Build history of the part. All positions in model axes, mm. A direction names the side the tool comes from. Round coordinates to 2 decimals unless told otherwise and drop trailing zeros. Write each loop counter-clockwise with the first axis right and the second up, starting at its lowest first coordinate (ties: lowest second). Pieces come first, ordered by that corner, then holes. Notation, with made-up numbers: M 7.5,57 L 39.5,57 A23 cw 39.5,81 Z; hole C 52,-35.75 d4. An arc over 180 degrees is marked long. Write item = value, one per line.
from build123d import *

# Parameters (mm, degrees)
PAD_DEPTH       = 20
SKETCH001_R     = 13
POCKET_DEPTH    = 18
SKETCH002_R     = 2.75
POCKET001_DEPTH = 74.863063
POCKET002_START = -20
SKETCH003_R     = 5
POCKET002_DEPTH = 50


with BuildPart() as part:
    # Sketch → Pad (new body)
    with BuildSketch(Plane.XY):
        with BuildLine():
            Line((0, 0), (0, 15))
            Line((24.254781, 65), (0, 15))
            ThreePointArc((55.745219, 65), (40, 74.862063), (24.254781, 65))
            Line((55.745219, 65), (80, 15))
            Line((80, 0), (80, 15))
            Line((0, 0), (80, 0))
        make_face()
    extrude(amount=PAD_DEPTH)

    # Sketch001 (on Face8 of Pad) → Pocket (cut)
    with BuildSketch(Plane.XY.offset(20)):
        with Locations((40, 57.362063)):
            Circle(SKETCH001_R)
    extrude(amount=-POCKET_DEPTH, mode=Mode.SUBTRACT)

    # Sketch002 (on Face7 of Pocket) → Pocket001 (cut, through all)
    with BuildSketch(Plane.XZ):
        with Locations((10, 10)):
            Circle(SKETCH002_R)
        with Locations((70, 10)):
            Circle(SKETCH002_R)
    extrude(amount=-POCKET001_DEPTH, mode=Mode.SUBTRACT)

    # Sketch003 → Pocket002 (cut)
    with BuildSketch(Plane.XZ.offset(POCKET002_START)):
        with Locations((70, 10)):
            Circle(SKETCH003_R)
        with Locations((10, 10)):
            Circle(SKETCH003_R)
    extrude(amount=-POCKET002_DEPTH, mode=Mode.SUBTRACT)


solid = part.part
1. Band-saw the part on D-D (x = 10). List the corners of the cut face in (y, z).
Responses:
outline = M 0,0 L 35.61,0 L 35.61,5 L 20,5 L 20,7.25 L 0,7.25 Z; M 0,12.75 L 20,12.75 L 20,15 L 35.61,15 L 35.61,20 L 0,20 Z
2. Mould opens along X. For faces 4 (the face through (0, 7, 10)), 5 (the face through (39, 0, 10)), 6 (the face through (65, 30, 10)) say: pulls with the +X half, pulls with the -X half, needs draft (parallel to the pull), parting line crosses it, or undercut.
Responses:
face_4 = pulls with the -X half
face_5 = needs draft
face_6 = undercut
3. Band-saw the part on B-B (x = 40). List the corners of the cut face in (y, z), plus the area to 3 significant figures.
Responses:
outline = M 0,0 L 74.86,0 L 74.86,20 L 70.36,20 L 70.36,2 L 44.36,2 L 44.36,20 L 0,20 Z
area = 1,030 mm²
4. Flat gauge pins, fed straight in: pin 1 (5 mm diameter, centred on y = 21.5, z = 5.5, fed in from -X); pin 2 (8 mm diameter, centred on y = 17, z = 6.5, fed in from +X); pin 3 (21 mm diameter, centred on x = 39.5, y = 59.5, fed in from +Z); pin 4 (1.5 mm diameter, centred on y = 33, z = 15.5, fed in from +X). Where does each tip first touch, or does it go through?
Responses:
pin_1 = 1.94
pin_2 = 80
pin_3 = 2
pin_4 = 71.63
5. Band-saw the part on A-A (z = 10). List the corners of the cut face in (x, y).
Responses:
outline = M 0,0 L 7.25,0 L 7.25,20 L 5,20 L 5,25.31 L 0,15 Z; M 12.75,0 L 67.25,0 L 67.25,20 L 65,20 L 65,45.92 L 55.75,65 A17.5 ccw 24.25,65 L 15,45.92 L 15,20 L 12.75,20 Z; M 72.75,0 L 80,0 L 80,15 L 75,25.31 L 75,20 L 72.75,20 Z; hole C 40,57.36 d26
6. Band-saw the part on C-C (y = 56). List the corners of the cut face in (x, z).
Responses:
outline = M 19.89,0 L 60.11,0 L 60.11,20 L 52.93,20 L 52.93,2 L 27.07,2 L 27.07,20 L 19.89,20 Z
7. Probe probe 1 along Z at (x, y) = (10, 5); probe 2 along Z at (x, y) = (10, 26.5); probe 3 along X at (y, z) = (55.5, 7.75). List the from-to ranges inside material, lowest first.
Responses:
probe_1 = 0 to 7.25, 12.75 to 20
probe_2 = 0 to 5, 15 to 20
probe_3 = 19.65 to 27.13, 52.87 to 60.35
8. Tool access for faces 1 (the face through (65.008, 45.906, 7.638)), 2 (the face through (27.013, 57.934, 11.126)), 3 (the face through (72.2, 20, 7.8)): list every direction of +Z, -Z, +X, -X, +Y, -Y with a clear straight run to the whole face (end or side of a thin tool).
Responses:
face_1 = +Z, -Z, +X, +Y
face_2 = +Z
face_3 = +Y
